```python
from build123d import *


with BuildPart() as part:
    # Sketch1 → Revolve1 (revolve)
    with BuildSketch(Plane(origin=(0, 0, 0), x_dir=(0, 0, -1), z_dir=(1, 0, 0))):
        with BuildLine():
            Line((0, 0), (-50.959835356, 0))
            Line((-50.959835356, 0), (-83.8211217, 0))
            Line((-83.8211217, 0), (-83.8211217, 75.282050808))
            Line((-83.8211217, 75.282050808), (-80.8211217, 73.55))
            Line((-80.8211217, 73.55), (-60.8211217, 73.55))
            Line((-60.8211217, 73.55), (-29.224979598, 35.895184138))
            ThreePointArc((-29.224979598, 35.895184138), (-25.002056634, 33.267714962), (-20.042663952, 33.643343571))
            ThreePointArc((-20.042663952, 33.643343571), (-10.179122164, 36.1760026), (0, 35.877187771))
            Line((0, 35.877187771), (0, 34.862194457))
            Line((0, 34.862194457), (0, 0))
        make_face()
    revolve(axis=Axis((0, 0, 0), (0, 0, 1)))


solid = part.part
```
Can you work these out from the model? Positions are in its coordinate system, mm. A direction names the side the tool comes from. Give positions to 0.01 mm unless a question says otherwise; leave off trailing zeros. Loops run counter-clockwise (first coordinate to the right, second up) from the corner with the lowest first, then second, coordinate; pieces in that order, holes last. Notation, with made-up numbers: M 36.5,31 L 77.5,31 A17 ccw 77.5,52 Z; hole C -28.75,-26.75 d10. An arc over 180 degrees is marked long. Answer in a Markdown table with one row per item.
1. Suppose I cut it at A-A on y = 0. Write out the boundary of the cut face in (x, z).
Taken from the geometry:
| item | result |
|---|---|
| outline | M -75.28,83.82 L -73.55,80.82 L -73.55,60.82 L -35.9,29.22 A8 cw -33.64,20.04 A36.4 ccw -35.88,0 L 35.88,0 A36.4 ccw 33.64,20.04 A8 cw 35.9,29.22 L 73.55,60.82 L 73.55,80.82 L 75.28,83.82 Z |
2. Suppose I cut it at B-B on z = 78. Write out the boundary of the cut face in (x, y), plus the area to 3 significant figures.
Taken from the geometry:
| item | result |
|---|---|
| outline | C 0,0 d147.1 |
| area | 17,000 mm² |
3. Which directions (+Z, -Z, +X, -X, +Y, -Y) give clear straight access to the entire face, cutting with the end or side of a thin tool? Please do faces 1 (the cylindrical face through (-22.092, 70.154, 70.681)), 2 (the flat face through (-1, 1, 83.821)).
Taken from the geometry:
| item | result |
|---|---|
| face 1 | -Z |
| face 2 | +Z, +X, -X, +Y, -Y |
4. For pin 1 Ø8 at (y, z) = (-53, 71.5) entering from +X; pin 2 Ø3 at (y, z) = (39.5, 11) entering from +X; pin 3 Ø1 at (y, z) = (-49, 66) entering from -X; pin 4 Ø12 at (x, z) = (45.5, 41) entering from -Y, each with a flat end and sliding along its axis, tell me the tip position at first contact or that it passes through.
Taken from the geometry:
| item | result |
|---|---|
| pin 1 | stops at x = 54.85 |
| pin 2 | passes through |
| pin 3 | stops at x = -55.29 |
| pin 4 | stops at y = -36.66 |
5. If I drill on line 1 along X through (y, z) = (-1.5, 76); line 2 along Y through (x, z) = (7.5, 4); line 3 along Z through (x, y) = (-38, 34), over which ranges is the centre line in solid material (lowest first)?
Taken from the geometry:
| item | result |
|---|---|
| line 1 | x = -73.53 to 73.53 |
| line 2 | y = -35.55 to 35.55 |
| line 3 | z = 41.89 to 83.82 |
6. Suppose I cut it at D-D on z = 8. Write out the boundary of the cut face in (x, y).
Taken from the geometry:
| item | result |
|---|---|
| outline | C 0,0 d72.71 |
